Check sheet for the modelled part. Datum: model origin and axes. Units: mm. Round coordinates to 2 decimals unless told otherwise and drop trailing zeros. Write each loop counter-clockwise with the first axis right and the second up, starting at its lowest first coordinate (ties: lowest second). Pieces come first, ordered by that corner, then holes. Notation, with made-up numbers: (34, 74) - (86, 74) arc R26 cw to (86, 110) - close; hole circle Ø11 at (-33, -17). An arc over 180 degrees is marked (long way). Answer as a JSON object with one key per item and string values. Group by question number.
Item 1: Release check for a two-part mould opening along X. For faces 1 (the cylindrical face through (-10.648, -13.887, 44.53)), 2 (the flat face through (-14, -7, 42.847)), 3 (the flat face through (-0.75, -12, 65)) record: pulls with the +X half, pulls with the -X half, needs draft (parallel to the pull), parting line crosses it, or undercut.
Item 2: Thickness scan on line 1 (X direction, y = 0, z = 44); line 2 (Y direction, x = -8, z = 60.5); line 3 (X direction, y = -1.5, z = 68). Record the ranges inside material, lowest first.
Item 3: Sectioned sample at C-C on z = 53. Record the boundary of the cut face in (x, y), plus the area to 3 significant figures.
Item 4: Sectioned sample at A-A on y = 0. Record the boundary of the cut face in (x, z), plus the area to 3 significant figures.
Item 5: Gauge pin test, flat ends, axial feed: P1, Ø5, axis at x = 11, z = 65, coming from the -Y side; P2, Ø1.5, axis at x = -3, y = 11.5, coming from the -Z side; P3, Ø1.5, axis at x = 7.5, z = 55, coming from the -Y side. Record the tip position at first contact, or that the pin passes through.
```python
from build123d import *

# Parameters (mm, degrees)
ESTRUSIONE_ESTRUSIONE1_REACH      = 63.48
ESTRUSIONE_ESTRUSIONE1_END_RADIUS = 18
ESTRUSIONE_ESTRUSIONE1_START      = -16.57
SCHIZZO3_R                        = 5


with BuildPart() as part:
    # Schizzo1 → Rivoluzione1 (revolve)
    with BuildSketch(Plane(origin=(0, 0, 0), x_dir=(0, 0, -1), z_dir=(1, 0, 0))):
        with BuildLine():
            Line((-46.259570065, 17.5), (-42.84743692, 17.5))
            Line((-42.84743692, 17.5), (-42.84743692, 15.5))
            Line((-42.84743692, 15.5), (-46.259570065, 15.5))
            ThreePointArc((-46.259570065, 15.5), (-51.319214322, 15.902531747), (-56.251566863, 17.1))
            ThreePointArc((-56.251566863, 17.1), (-58.035417815, 17.58636227), (-59.85975099, 17.887162773))
            ThreePointArc((-59.85975099, 17.887162773), (-71.267974414, 11.995381335), (-75.84743692, 0))
            Line((-75.84743692, 0), (-77.84743692, 0))
            ThreePointArc((-77.84743692, 0), (-72.683984385, 13.411817897), (-59.85975099, 19.898507283))
            ThreePointArc((-59.85975099, 19.898507283), (-57.719038516, 19.56405813), (-55.627067063, 19))
            ThreePointArc((-55.627067063, 19), (-51.002986556, 17.877373513), (-46.259570065, 17.5))
        make_face()
    revolve(axis=Axis((0, 0, 77.84743692), (0, 0, -1)))

    # Estrusione-Estrusione1: up to this sphere (the profile starts inside it)
    estrusione_estrusione1_end = Location((0, 0, 57.84743692)) * Sphere(ESTRUSIONE_ESTRUSIONE1_END_RADIUS, mode=Mode.PRIVATE)
    # Schizzo3 → Estrusione-Estrusione1 (add, up to the surface)
    with BuildSketch(Plane(origin=(0, 0, 42.84743692), x_dir=(-1, 0, 0), z_dir=(0, 0, -1)).offset(ESTRUSIONE_ESTRUSIONE1_START), mode=Mode.PRIVATE) as estrusione_estrusione1_sk1:
        with BuildLine():
            Line((-17.87143229, -0.75), (-7.462405778, -0.75))
            ThreePointArc((-7.462405778, -0.75), (-5.303300859, -5.303300859), (-0.75, -7.462405778))
            Line((-0.75, -7.462405778), (-0.75, -17.87143229))
            ThreePointArc((-0.75, -17.87143229), (0, -17.887162773), (0.75, -17.87143229))
            Line((0.75, -17.87143229), (0.75, -7.462405778))
            ThreePointArc((0.75, -7.462405778), (5.303300859, -5.303300859), (7.462405778, -0.75))
            Line((7.462405778, -0.75), (17.87143229, -0.75))
            ThreePointArc((17.87143229, -0.75), (17.887162773, 0), (17.87143229, 0.75))
            Line((17.87143229, 0.75), (7.462405778, 0.75))
            ThreePointArc((7.462405778, 0.75), (5.303300859, 5.303300859), (0.75, 7.462405778))
            Line((0.75, 7.462405778), (0.75, 17.87143229))
            ThreePointArc((0.75, 17.87143229), (0, 17.887162773), (-0.75, 17.87143229))
            Line((-0.75, 17.87143229), (-0.75, 7.462405778))
            ThreePointArc((-0.75, 7.462405778), (-5.303300859, 5.303300859), (-7.462405778, 0.75))
            Line((-7.462405778, 0.75), (-17.87143229, 0.75))
            ThreePointArc((-17.87143229, 0.75), (-17.887162773, 0), (-17.87143229, -0.75))
        make_face()
        Circle(SCHIZZO3_R, mode=Mode.SUBTRACT)
    estrusione_estrusione1_tool1 = extrude(estrusione_estrusione1_sk1.sketch, amount=-ESTRUSIONE_ESTRUSIONE1_REACH, mode=Mode.PRIVATE) & estrusione_estrusione1_end
    add(estrusione_estrusione1_tool1.solids().sort_by_distance((12.666919, -0.244075, 59.417437))[0])


solid = part.part
```
Completed:
{
 "1": {"face 1": "parting line crosses it", "face 2": "needs draft", "face 3": "undercut"},
 "2": {"line 1": "-17.5 to -15.5, 15.5 to 17.5", "line 2": "-18.14 to -15.9, -0.75 to 0.75, 15.9 to 18.14", "line 3": "-17.17 to -14.79, -7.35 to -4.77, 4.77 to 7.35, 14.79 to 17.17"},
 "3": {"outline": "circle Ø36.53 at (0, 0); hole circle Ø32.44 at (0, 0)", "area": "222 mm²"},
 "4": {"outline": "(-19.9, 59.86) arc R20 ccw to (-19, 55.63) arc R30 cw to (-17.5, 46.26) - (-17.5, 42.85) - (-15.5, 42.85) - (-15.5, 46.26) arc R32 ccw to (-17.1, 56.25) arc R18 cw to (-17.83, 59.42) - (-5, 59.42) - (-5, 75.14) arc R18 cw to (5, 75.14) - (5, 59.42) - (17.83, 59.42) arc R18 cw to (17.1, 56.25) arc R32 ccw to (15.5, 46.26) - (15.5, 42.85) - (17.5, 42.85) - (17.5, 46.26) arc R30 cw to (19, 55.63) arc R20 ccw to (19.9, 59.86) arc R20 ccw to start", "area": "471 mm²"},
 "5": {"P1": "y = -16.95", "P2": "z = 70.67", "P3": "y = -17.64"}
}
